```python
from build123d import *

# Parameters (mm, degrees)
BOSS_EXTRUDE1_DEPTH = 20
SKETCH6_R           = 1.6
CUT_EXTRUDE4_DEPTH  = 30.732137495
SKETCH7_R           = 2.7
CUT_EXTRUDE5_DEPTH  = 28.079952174
FILLET4_R           = 1
FILLET5_R           = 0.5
CUT_EXTRUDE6_DEPTH  = 10
CUT_EXTRUDE7_DEPTH  = 10
FILLET6_R           = 1.5
CUT_EXTRUDE8_DEPTH  = 26
SKETCH11_R          = 1.6
CUT_EXTRUDE9_DEPTH  = 26
SKETCH12_R          = 3.6
CUT_EXTRUDE10_DEPTH = 10
CUT_EXTRUDE13_DEPTH = 25
SKETCH14_R          = 4.5
CUT_EXTRUDE14_DEPTH = 10


# Read off the part's stored shape, not the designer's step: Mirror1
with BuildPart() as part:
    # Sketch1 → Boss-Extrude1 (new body)
    with BuildSketch(Plane.XY):
        Polygon((0, 0), (0, 15.556349186), (15.556349186, 0), align=None)
    extrude(amount=BOSS_EXTRUDE1_DEPTH)

    # Sketch6 → Cut-Extrude4 (cut, through all)
    with BuildSketch(Plane.ZY):
        with Locations((16.335044769, 3.48)):
            Circle(SKETCH6_R)
        with Locations((3.664955231, 3.48)):
            Circle(SKETCH6_R)
    extrude(amount=-CUT_EXTRUDE4_DEPTH, mode=Mode.SUBTRACT)

    # Sketch7 → Cut-Extrude5 (cut, through all)
    with BuildSketch(Plane.ZY.offset(-6)):
        with Locations((16.335044769, 3.48)):
            Circle(SKETCH7_R)
        with Locations((3.664955231, 3.48)):
            Circle(SKETCH7_R)
    extrude(amount=-CUT_EXTRUDE5_DEPTH, mode=Mode.SUBTRACT)

    # Fillet4
    fillet4_edges = [part.edges().sort_by_distance(p)[0] for p in [
        (0, 0, 10),
    ]]
    fillet(fillet4_edges, radius=FILLET4_R)

    # Fillet5
    # the kernel refuses this fillet: 0.5 mm, written as the material it takes off along each edge
    with BuildSketch(Plane(origin=(15.556349186, 0, -3.017766953), x_dir=(-0.7071067811865474, 0.7071067811865477, 0), z_dir=(0, 0, 1)), Plane(origin=(0, 15.556349186, -3.017766953), x_dir=(0, -1, 0), z_dir=(0, 0, 1))) as fillet5_piece_1:
        with BuildLine():
            CenterArc((FILLET5_R * 2.41421356237, FILLET5_R), FILLET5_R, 135, 135)
            Line((FILLET5_R * 1.70710678119, FILLET5_R * 1.70710678119), (0, 0))
            Line((0, 0), (FILLET5_R * 2.41421356237, 0))
        make_face()
    extrude(amount=26.035533906, mode=Mode.SUBTRACT)

    # Sketch8 → Cut-Extrude6 (cut)
    with BuildSketch(Plane(origin=(7.778174593, 7.778174593, 0), x_dir=(0, 0, -1), z_dir=(0.7071067811865477, 0.7071067811865475, 0))):
        Polygon((-20, -12.333051339), (0, -12.333051339), (0.012190886, -3.93058749), (-20, -3.93058749), align=None)
    extrude(amount=-CUT_EXTRUDE6_DEPTH, mode=Mode.SUBTRACT)

    # Sketch9 → Cut-Extrude7 (cut)
    with BuildSketch(Plane(origin=(7.778174593, 7.778174593, 0), x_dir=(0, 0, -1), z_dir=(0.7071067811865477, 0.7071067811865475, 0))):
        Polygon((-11.323221056, 10.808771842), (0, 5.528667149), (0, 10.808771842), align=None)
    extrude(amount=-CUT_EXTRUDE7_DEPTH, mode=Mode.SUBTRACT)

    # Fillet6
    fillet6_edges = [part.edges().sort_by_distance(p)[0] for p in [
        (8.058104899, 2.499414762, 0),
        (1.934408281, 9.753124344, 0),
    ]]
    fillet(fillet6_edges, radius=FILLET6_R)

    # Mirror1: part across plane


with BuildPart() as part_1:
    add(part.part)
    add(part.part.mirror(Plane(origin=(0, 15.556349186, 20), x_dir=(0, 0, 1), z_dir=(-0.7071067811865476, -0.7071067811865476, 0))))

    # Sketch10 → Cut-Extrude8 (cut)
    with BuildSketch(Plane.XY.offset(20)):
        Polygon((0.853553391, 14.702795796), (12.695020556, 2.86132863), (4.968641211, -4.865050714), (-9.455036557, 9.558627055), (-1.728657213, 17.285006399), align=None)
    extrude(amount=-CUT_EXTRUDE8_DEPTH, mode=Mode.SUBTRACT)

    # Sketch11 → Cut-Extrude9 (cut)
    with BuildSketch(Plane(origin=(7.778174593, 7.778174593, 0), x_dir=(0, 0, 1), z_dir=(-0.7071067811865477, -0.7071067811865475, 0))):
        with Locations(Location((10.089715554, 3.018295217, 0), (0, 0, 270))):
            Circle(SKETCH11_R)
    extrude(amount=-CUT_EXTRUDE9_DEPTH, mode=Mode.SUBTRACT)

    # Sketch12 → Cut-Extrude10 (cut)
    with BuildSketch(Plane(origin=(11.313708499, 11.313708499, 0), x_dir=(-0.7071067811865475, 0.7071067811865477, 0), z_dir=(-0.7071067811865477, -0.7071067811865475, 0))):
        with Locations((3.018295217, -10.089715554)):
            Circle(SKETCH12_R)
    extrude(amount=-CUT_EXTRUDE10_DEPTH, mode=Mode.SUBTRACT)

    # Sketch13 → Cut-Extrude13 (cut)
    with BuildSketch(Plane.XY.offset(20)):
        Polygon((15.86082052, 10.302130384), (8.59176281, 10.302130384), (6.922990806, 8.63335838), (10.557519661, 4.998829525), align=None)
    extrude(amount=-CUT_EXTRUDE13_DEPTH, mode=Mode.SUBTRACT)

    # Sketch14 → Cut-Extrude14 (cut)
    with BuildSketch(Plane.XZ.offset(-10.302130384)):
        with Locations((12.076349186, 16.335044769)):
            Circle(SKETCH14_R)
        with Locations((12.076349186, 3.664955231)):
            Circle(SKETCH14_R)
    extrude(amount=CUT_EXTRUDE14_DEPTH, mode=Mode.SUBTRACT)


solid = part_1.part
```
Check sheet for the modelled part. Datum: model origin and axes. Units: mm. A direction names the side the tool comes from. Coordinates: 2 decimals unless noted, no trailing zeros. Write each loop counter-clockwise with the first axis right and the second up, starting at its lowest first coordinate (ties: lowest second). Pieces come first, ordered by that corner, then holes. Notation, with made-up numbers: M 45.5,-35.5 L 68.5,-35.5 A23 cw 68.5,-5.5 Z; hole C -26,45.5 d7. An arc over 180 degrees is marked long. Write item = value, one per line. Start each with the question number.
1. Thickness scan on probe 1 along Z at (x, y) = (12.75, 15); probe 2 along Y at (x, z) = (14.75, 2.5); probe 3 along X at (y, z) = (11.75, 8.75). Record the ranges inside material, lowest first.
2. Sectioned sample at A-A (z = 4). Record the cut outline in (x, y), then the cut area to 3 significant figures.
3. Sectioned sample at D-D (y = 13). State how many separate pieces and enclosed holes the cut face has, then the cut area to 3 significant figures.
4. Go/stop test with flat-tipped pins: pin 1 (3 mm diameter, centred on y = 9.5, z = 12, fed in from -X); pin 2 (1 mm diameter, centred on x = 11.5, z = 7.5, fed in from +Y); pin 3 (4 mm diameter, centred on x = 12.08, z = 3.66, fed in from +Y). Record where each tip stops, or that it passes through.
5. Tool access check on faces 1 (the cylindrical face through (13.64, 12.97, 15.99)), 2 (the cylindrical face through (7.577, 9.855, 3.708)). Record the directions out of +Z, -Z, +X, -X, +Y, -Y that give a thin tool (end or side, any length) a straight path to the whole face; none if there is none.
6. Sectioned sample at C-C (z = 17.25). Record the cut outline in (x, y).
7. Mould release check, pull along X, two halves, no side actions. Record for faces 3 (the flat face through (3.846, 11.711, 10.14)), 4 (the cylindrical face through (8, 11.05, 11.44)), 5 (the cylindrical face through (15.256, 15.271, 12.362)): pulls with the +X half, pulls with the -X half, needs draft (parallel to the pull), parting line crosses it, or undercut.
8. Sectioned sample at B-B (z = 6.25). Record the cut outline in (x, y), then the cut area to 3 significant figures.
The answers:
q1.probe_1 = 0 to 2.21, 5.12 to 6.78, 13.39 to 14.88, 17.79 to 20
q1.probe_2 = 10.3 to 15.54
q1.probe_3 = 3.81 to 6.24, 8.72 to 10.88, 12.21 to 15.56
q2.outline = M 2.55,13.01 L 6.92,8.63 L 7.59,9.3 L 7.59,10.3 L 10.51,10.3 L 10.51,15.56 L 5.1,15.56 Z; M 13.64,10.3 L 15.56,10.3 L 15.56,14.56 A1 ccw 14.56,15.56 L 13.64,15.56 Z
q2.area = 47.1 mm²
q3.separate_pieces = 1
q3.enclosed_holes = 3
q3.area = 208 mm²
q4.pin_1 = 4.56
q4.pin_2 = 13.26
q4.pin_3 = 15.56
q5.face_1 = +Y, -Y
q5.face_2 = +X, -Y
q6.outline = M 0.85,14.7 L 6.92,8.63 L 7.67,9.38 L 7.67,10.3 L 10.76,10.3 L 10.76,15.56 L 1.21,15.56 A0.5 ccw Z; M 13.39,10.3 L 15.56,10.3 L 15.56,14.56 A1 ccw 14.56,15.56 L 13.39,15.56 Z
q7.face_3 = pulls with the -X half
q7.face_4 = undercut
q7.face_5 = pulls with the +X half
q8.outline = M 1.81,13.75 L 6.92,8.63 L 8.39,10.1 L 8.39,10.3 L 15.56,10.3 L 15.56,14.56 A1 ccw 14.56,15.56 L 3.62,15.56 Z
q8.area = 67.2 mm²
